Build history of the part. All positions in model axes, mm. Face numbers are marked on the shaded views. A direction names the side the tool comes from. Give positions to 0.01 mm unless a question says otherwise; leave off trailing zeros. Loops run counter-clockwise (first coordinate to the right, second up) from the corner with the lowest first, then second, coordinate; pieces in that order, holes last. Notation, with made-up numbers: (32.25, 8) -> (76.25, 8) arc R30 cw to (76.25, 36) -> close; hole circle Ø4 at (-38, 76.25). An arc over 180 degrees is marked (long way). Answer as a JSON object with one key per item and string values. Group by question number.
Q1. Band-saw the part on B-B, the plane y = 13. Write the cut outline in (x, z), plus the area to 3 significant figures.
Q2. Wall check: probe 1 along Y at (x, z) = (0, 8); probe 2 along X at (y, z) = (125, -6.65); probe 3 along Z at (x, y) = (-30, 10). Give the ranges that are in metal, low to high. Write a range as from..to.
Q3. Two-plate mould, pull along X, no slides. Class the marked faces 1, 2, 3 and 4: pulls with the +X half, pulls with the -X half, needs draft (parallel to the pull), parting line crosses it, or undercut.
Q4. Tool access for the marked faces 5, 6 and 7: list every direction of +Z, -Z, +X, -X, +Y, -Y with a clear straight run to the whole face (end or side of a thin tool).
Q5. Band-saw the part on A-A, the plane x = 0. Write the cut outline in (y, z).
Q6. Drop flat-ended pins along their axis: pin 1 (2.5 mm diameter, centred on x = -22, z = -4, fed in from +Y); pin 2 (4 mm diameter, centred on y = 87.5, z = 4.5, fed in from +X); pin 3 (1 mm diameter, centred on y = 88, z = -9.5, fed in from -X); pin 4 (3 mm diameter, centred on x = 27, y = 37, fed in from +Z). Give the stop position or say it passes through.
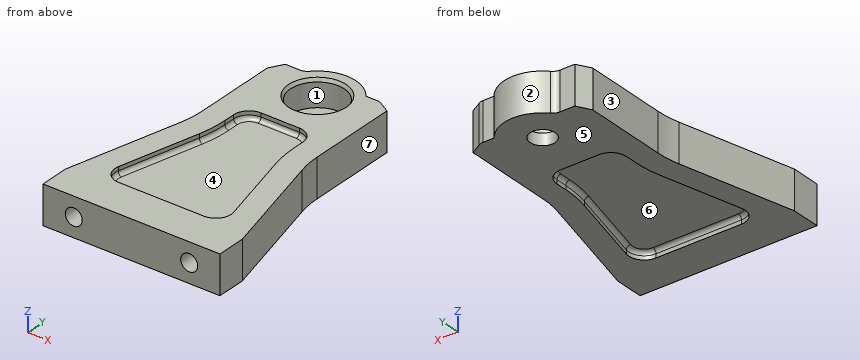
from build123d import *
from OCP.BRepFilletAPI import BRepFilletAPI_MakeChamfer

# Parameters (mm, degrees)
SKETCH1_R                   = 6.5
BOSS_EXTRUDE1_DEPTH         = 10
SKETCH2_R                   = 14
CUT_EXTRUDE1_DEPTH          = 14
CHAMFER1_SIZE               = 1
CHAMFER1_SIZE2              = 1.732050808
CHAMFER2_SIZE               = 4
CHAMFER2_SIZE2              = 6.92820323
FILLET1_R                   = 5
CUT_EXTRUDE2_DEPTH          = 4
FILLET2_R                   = 2
FILLET2_OF_MIRROR1_R        = 2
M10X1_25_TAPPED_HOLE1_D     = 8.8
M10X1_25_TAPPED_HOLE1_DEPTH = 20
M10X1_25_TAPPED_HOLE1_TIP   = 2.643786724


with BuildPart() as part:
    # Sketch1 → Boss-Extrude1 (new, symmetric)
    with BuildSketch(Plane.XY):
        with BuildLine():
            Line((-46, 0), (46, 0))
            Line((46, 0), (46, 15))
            Line((46, 15), (31.449256053, 74.112397284))
            ThreePointArc((31.449256053, 74.112397284), (30.363636327, 80.044097084), (30, 86.06334964))
            Line((30, 86.06334964), (30, 137))
            Line((30, 137), (16, 137))
            ThreePointArc((16, 137), (0, 145), (-16, 137))
            Line((-16, 137), (-30, 137))
            Line((-30, 137), (-30, 86.06334964))
            ThreePointArc((-30, 86.06334964), (-30.363636327, 80.044097084), (-31.449256053, 74.112397284))
            Line((-31.449256053, 74.112397284), (-46, 15))
            Line((-46, 15), (-46, 0))
        make_face()
        with Locations((0, 125)):
            Circle(SKETCH1_R, mode=Mode.SUBTRACT)
    extrude(amount=BOSS_EXTRUDE1_DEPTH, both=True)

    # Sketch2 → Cut-Extrude1 (cut)
    with BuildSketch(Plane.XY.offset(10)):
        with Locations((0, 125)):
            Circle(SKETCH2_R)
    extrude(amount=-CUT_EXTRUDE1_DEPTH, mode=Mode.SUBTRACT)

    # Chamfer1
    chamfer1_edges = [part.edges().sort_by_distance(p)[0] for p in [
        (-14, 125, 10),
    ]]
    chamfer1_side = [part.faces().sort_by_distance(p)[0] for p in [
        (0, 59.441099991, 10),
    ]]
    chamfer(chamfer1_edges, length=CHAMFER1_SIZE, length2=CHAMFER1_SIZE2, reference=chamfer1_side[0])

    # Chamfer2: one chamfer whose edges measure the first distance from different faces: ONE call of the kernel's chamfer builder (chamfer() names one face for all edges)
    chamfer2_edges_1 = [part.edges().sort_by_distance(p)[0] for p in [
        (-30, 137, 0),
    ]]
    chamfer2_side_1 = [part.faces().sort_by_distance(p)[0] for p in [
        (-23, 137, 0),
    ]]
    chamfer2_edges_2 = [part.edges().sort_by_distance(p)[0] for p in [
        (30, 137, 0),
    ]]
    chamfer2_side_2 = [part.faces().sort_by_distance(p)[0] for p in [
        (30, 111.53167482, 0),
    ]]
    chamfer2 = BRepFilletAPI_MakeChamfer(part.part.solid().wrapped)
    for e in chamfer2_edges_1:
        chamfer2.Add(CHAMFER2_SIZE, CHAMFER2_SIZE2, e.wrapped, chamfer2_side_1[0].wrapped)  # the first distance lies on this face
    for e in chamfer2_edges_2:
        chamfer2.Add(CHAMFER2_SIZE, CHAMFER2_SIZE2, e.wrapped, chamfer2_side_2[0].wrapped)  # the first distance lies on this face
    add(Compound.cast(chamfer2.Shape()), mode=Mode.REPLACE)

    # Fillet1
    fillet1_edges = [part.edges().sort_by_distance(p)[0] for p in [
        (-16, 137, 0),
        (23.07179677, 137, 0),
    ]]
    fillet(fillet1_edges, radius=FILLET1_R)

    # Sketch4 → Cut-Extrude2 (cut)
    with BuildSketch(Plane.XY.offset(10)):
        with BuildLine():
            ThreePointArc((-19.797077506, 71.244168718), (-18.450909046, 78.59947647), (-18, 86.06334964))
            Line((-18, 86.06334964), (-18, 92))
            ThreePointArc((-18, 92), (-15.656854249, 97.656854249), (-10, 100))
            Line((-10, 100), (10, 100))
            ThreePointArc((10, 100), (15.656854249, 97.656854249), (18, 92))
            Line((18, 92), (18, 86.06334964))
            ThreePointArc((18, 86.06334964), (18.450909046, 78.59947647), (19.797077506, 71.244168718))
            Line((19.797077506, 71.244168718), (29.971112298, 29.912152377))
            ThreePointArc((29.971112298, 29.912152377), (28.49970745, 23.065287193), (22.202993266, 20))
            Line((22.202993266, 20), (-22.202993266, 20))
            ThreePointArc((-22.202993266, 20), (-28.49970745, 23.065287193), (-29.971112298, 29.912152377))
            Line((-29.971112298, 29.912152377), (-19.797077506, 71.244168718))
        make_face()
    cut_extrude2 = extrude(amount=-CUT_EXTRUDE2_DEPTH, mode=Mode.SUBTRACT)

    # Fillet2
    fillet2_edges = [part.edges().sort_by_distance(p)[0] for p in [
        (-18, 89.03167482, 6),
        (-15.656854249, 97.656854249, 6),
        (18, 89.03167482, 6),
        (24.884094902, 50.578160548, 6),
        (28.49970745, 23.065287193, 6),
        (0, 20, 6),
        (-24.884094902, 50.578160548, 6),
        (-18.450909046, 78.59947647, 6),
        (0, 100, 6),
        (15.656854249, 97.656854249, 6),
        (18.450909046, 78.59947647, 6),
        (-28.49970745, 23.065287193, 6),
    ]]
    fillet(fillet2_edges, radius=FILLET2_R)

    # Mirror1: Cut-Extrude2 across plane
    add(cut_extrude2.mirror(Plane.XY), mode=Mode.SUBTRACT)

    # Fillet2 of Mirror1
    fillet2_of_mirror1_edges = [part.edges().sort_by_distance(p)[0] for p in [
        (-18, 89.03167482, -6),
        (-15.656854249, 97.656854249, -6),
        (18, 89.03167482, -6),
        (24.884094902, 50.578160548, -6),
        (28.49970745, 23.065287193, -6),
        (0, 20, -6),
        (-24.884094902, 50.578160548, -6),
        (-18.450909046, 78.59947647, -6),
        (0, 100, -6),
        (15.656854249, 97.656854249, -6),
        (18.450909046, 78.59947647, -6),
        (-28.49970745, 23.065287193, -6),
    ]]
    fillet(fillet2_of_mirror1_edges, radius=FILLET2_OF_MIRROR1_R)

    # M10x1.25 Tapped Hole1
    with Locations(Plane(origin=(0, 0, 0), x_dir=(-1, 0, 0), z_dir=(0, -1, 0))):
        with Locations((-30, 0), (30, 0)):
            Hole(M10X1_25_TAPPED_HOLE1_D / 2, depth=M10X1_25_TAPPED_HOLE1_DEPTH)
            with Locations((0, 0, -(M10X1_25_TAPPED_HOLE1_DEPTH + M10X1_25_TAPPED_HOLE1_TIP / 2))):  # 118° drill point
                Cone(0, M10X1_25_TAPPED_HOLE1_D / 2, M10X1_25_TAPPED_HOLE1_TIP, mode=Mode.SUBTRACT)


solid = part.part
Worked answers:
{
 "1": {"outline": "(-46, -10) -> (46, -10) -> (46, 10) -> (-46, 10) -> close; hole circle Ø8.8 at (-30, 0); hole circle Ø8.8 at (30, 0)", "area": "1,720 mm2"},
 "2": {"probe 1": "0..20, 100..111, 139..145", "probe 2": "-30..-6.5, 6.5..30", "probe 3": "-10..-4.4, 4.4..10"},
 "3": {"face 1": "undercut", "face 2": "parting line crosses it", "face 3": "pulls with the -X half", "face 4": "undercut"},
 "4": {"face 5": "-Z, +X, -X, +Y, -Y", "face 6": "-Z", "face 7": "+Z, -Z, +X, +Y"},
 "5": {"outline": "(0, -10) -> (20, -10) -> (20, -8) arc R2 cw to (22, -6) -> (98, -6) arc R2 cw to (100, -8) -> (100, -10) -> (118.5, -10) -> (118.5, -4) -> (111, -4) -> (111, 8.27) -> (110, 10) -> (100, 10) -> (100, 8) arc R2 cw to (98, 6) -> (22, 6) arc R2 cw to (20, 8) -> (20, 10) -> (0, 10) -> close; (131.5, -10) -> (145, -10) -> (145, 10) -> (140, 10) -> (139, 8.27) -> (139, -4) -> (131.5, -4) -> close"},
 "6": {"pin 1": "y = 137", "pin 2": "x = 30", "pin 3": "x = -30", "pin 4": "z = 10"}
}
